from build123d import *

# Parameters (mm, degrees)
SKETCH_1_R      = 9
SKETCH_1_R_2    = 0.75
EXTRUDE_1_DEPTH = 1.5
SKETCH_2_R      = 3
SKETCH_2_R_2    = 2
EXTRUDE_2_DEPTH = 2
EXTRUDE_START   = 1
SKETCH_3_R      = 3
SKETCH_3_R_2    = 2
EXTRUDE_3_DEPTH = 1


with BuildPart() as part:
    # 草图1 → 凸台-拉伸1 (new body)
    with BuildSketch(Plane.XY):
        Circle(SKETCH_1_R)
        Circle(SKETCH_1_R_2, mode=Mode.SUBTRACT)
    extrude(amount=EXTRUDE_1_DEPTH)

    # 草图2 → 凸台-拉伸2 (add)
    with BuildSketch(Plane.XY.offset(1.5)):
        Circle(SKETCH_2_R)
        Circle(SKETCH_2_R_2, mode=Mode.SUBTRACT)
    extrude(amount=EXTRUDE_2_DEPTH)

    # 草图3 → 凸台-拉伸3 (add)
    with BuildSketch(Plane(origin=(0, 0, 0), x_dir=(-1, 0, 0), z_dir=(0, 0, -1)).offset(EXTRUDE_START)):
        with Locations(Location((0, 0, 0), (0, 0, 180))):
            Circle(SKETCH_3_R)
        with Locations(Location((0, 0, 0), (0, 0, 180))):
            Circle(SKETCH_3_R_2, mode=Mode.SUBTRACT)
    extrude(amount=-EXTRUDE_3_DEPTH)


solid = part.part
The listing builds one solid part. Answer for the finished solid, in the listing's coordinates (mm). A direction names the side the tool comes from. Round coordinates to 2 decimals unless told otherwise and drop trailing zeros. Loops run counter-clockwise (first coordinate to the right, second up) from the corner with the lowest first, then second, coordinate; pieces in that order, holes last. Notation, with made-up numbers: M 19,47.25 L 24,47.25 A30 ccw 24,79.25 Z; hole C 88.25,85.5 d7. An arc over 180 degrees is marked long. Return JSON: item names as keys, results as strings.
Q1. Which of the six approach directions +Z, -Z, +X, -X, +Y, -Y give full straight-line access (tool end or side, diameter ignored) to faces 4 (the face through (1, 0, 1.5)), 5 (the face through (-0.75, 0.03, 0.74)), 6 (the face through (1, 0, 0))?
Results list:
{"face 4": "+Z", "face 5": "+Z, -Z", "face 6": "-Z"}
Q2. Find section D-D, the plane y = 7.75. Determine the outline of the cut face in (x, z).
Results list:
{"outline": "M -4.58,0 L 4.58,0 L 4.58,1.5 L -4.58,1.5 Z"}
Q3. Each of these flat-tipped pins is pushed along its axis until it touches: pin 1 Ø3 at (x, y) = (0, 0) entering from +Z; pin 2 Ø1 at (y, z) = (-3.5, 1.5) entering from +X; pin 3 Ø3.5 at (x, y) = (0, 0) entering from -Z. Where does it stop, or does it pass through?
Results list:
{"pin 1": "stops at z = 1.5", "pin 2": "stops at x = 8.49", "pin 3": "stops at z = 0"}
Q4. Find section C-C, the plane z = 1.15. Determine the outline of the cut face in (x, y), plus the area to 3 significant figures.
Results list:
{"outline": "C 0,0 d18; hole C 0,0 d1.5", "area": "253 mm2"}
Q5. The mould has two halves that part along X. Classify faces 1 (the face through (-3, 0, 2)), 2 (the face through (0, -2, 2)), 3 (the face through (0, -4, 1.5)): released by +X, released by -X, zero draft, split by the parting line, or undercut.
Results list:
{"face 1": "split by the parting line", "face 2": "undercut", "face 3": "zero draft"}
Q6. Find section A-A, the plane x = 0. Determine the outline of the cut face in (y, z), plus the area to 4 significant figures.
Results list:
{"outline": "M -9,0 L -3,0 L -3,-1 L -2,-1 L -2,0 L -0.75,0 L -0.75,1.5 L -2,1.5 L -2,3.5 L -3,3.5 L -3,1.5 L -9,1.5 Z; M 0.75,0 L 2,0 L 2,-1 L 3,-1 L 3,0 L 9,0 L 9,1.5 L 3,1.5 L 3,3.5 L 2,3.5 L 2,1.5 L 0.75,1.5 Z", "area": "30.75 mm2"}
Q7. Find the intervals of material crossed by line 1 along Y through (x, z) = (0, -0.25); line 2 along Y through (x, z) = (0, 1.15); line 3 along Z through (x, y) = (-5.5, -4), in increasing order. Write a range as from..to.
Results list:
{"line 1": "y = -3..-2, 2..3", "line 2": "y = -9..-0.75, 0.75..9", "line 3": "z = 0..1.5"}
